Could you check a few things on this model? Use its own coordinates, in mm. A direction names the side the tool comes from. Give positions to 0.01 mm unless a question says otherwise; leave off trailing zeros. Write each loop counter-clockwise with the first axis right and the second up, starting at its lowest first coordinate (ties: lowest second). Pieces come first, ordered by that corner, then holes. Notation, with made-up numbers: M -16.75,49 L 9.25,49 A8 cw 9.25,61 Z; hole C 17.25,-9 d11. An arc over 180 degrees is marked long. Answer as CSV lines item,"result". Start each with the question number.
from build123d import *

# Parameters (mm, degrees)
F0_W       = 30
F0_H       = 50
F0_R       = 7.5
F0_H_2     = 5
F1_DEPTH   = 10
F2_W       = 30
F2_H       = 5
F1_FACE1_W = 30
F1_FACE1_H = 55
F1_FACE1_R = 7.5
F3_DEPTH   = 5


# Not quite as in the source:
# - a feature names something its author has since deleted; it is built from what else it names


with BuildPart() as f1:
    # F0 (on Front) → F1 (new body)
    with BuildSketch(Plane.XZ):
        Rectangle(F0_W, F0_H)
        with Locations((0, -1)):
            Circle(F0_R, mode=Mode.SUBTRACT)
        with Locations((0, -27.5)):
            Rectangle(F0_W, F0_H_2)
    extrude(amount=F1_DEPTH)

    # F2 (on face) + F1_face1 (on face) → F3 (join)
    with BuildSketch(Plane(origin=(0, 0, 0), x_dir=(-1, 0, 0), z_dir=(0, 1, 0))):
        with Locations((0, -27.5)):
            Rectangle(F2_W, F2_H)
    with BuildSketch(Plane(origin=(0, -10, -2.6799188927), x_dir=(1, 0, 0), z_dir=(0, -1, 0))):
        with Locations((0, 0.1799188927)):
            Rectangle(F1_FACE1_W, F1_FACE1_H)
        with Locations((0, 1.6799188927)):
            Circle(F1_FACE1_R, mode=Mode.SUBTRACT)
    extrude(amount=F3_DEPTH, dir=(0, 1, 0))


solid = f1.part
1. Imagine slicing it at D-D, the plane z = 14.5. Please give me the cut outline in (x, y).
2. Thinking about a two-plate mould opening in Z: for faces 3 (the flat face through (0, 5, -27)), 4 (the flat face through (0, -3, -30)), 5 (the cylindrical face through (-7.493, -4.93, -0.67)), which applies, pulls with the +Z half, pulls with the -Z half, needs draft (parallel to the pull), parting line crosses it, or undercut?
3. Imagine slicing it at B-B, the plane z = -1. Please give me the cut outline in (x, y), plus the area to 3 significant figures.
4. Imagine slicing it at A-A, the plane x = 0. Please give me the cut outline in (y, z).
5. Imagine slicing it at C-C, the plane y = -3. Please give me the cut outline in (x, z), plus the area to 3 significant figures.
6. Please list where these lines run through material, in increasing order: line 1 (Z direction, x = 0, y = -7.5); line 2 (Y direction, x = 9.5, z = 12.5); line 3 (Z direction, x = -12.25, y = 3.75).
7. On a 3-axis mill with a long thin cutter (end or side, diameter ignored), from which of +Z, -Z, +X, -X, +Y, -Y can I reach the whole of each face in a straight line? I mean faces 1 (the flat face through (0, 2, -25)), 2 (the flat face through (-4, -10, -8)). Say none if no direction works.
8. Will this pin go through, and if not, where does the flat tip stop? P1, Ø10, axis at x = 1.5, z = -17, coming from the +Y side.
Solutions:
1,outline,"M -15,-10 L 15,-10 L 15,0 L -15,0 Z"
2,face 3,"needs draft"
2,face 4,"pulls with the -Z half"
2,face 5,"undercut"
3,outline,"M -15,-10 L -7.5,-10 L -7.5,0 L -15,0 Z; M 7.5,-10 L 15,-10 L 15,0 L 7.5,0 Z"
3,area,"150 mm²"
4,outline,"M -10,-30 L 5,-30 L 5,-25 L 0,-25 L 0,-8.5 L -10,-8.5 Z; M -10,6.5 L 0,6.5 L 0,25 L -10,25 Z"
5,outline,"M -15,-30 L 15,-30 L 15,25 L -15,25 Z; hole C 0,-1 d15"
5,area,"1,470 mm²"
6,line 1,"-30 to -8.5, 6.5 to 25"
6,line 2,"-10 to 0"
6,line 3,"-30 to -25"
7,face 1,"+Z, +X, -X, +Y"
7,face 2,"+Z, -Z, +X, -X, -Y"
8,P1,"y = 0"
